Could you check a few things on this model? Use its own coordinates, in mm. Face numbers are marked on the shaded views. A direction names the side the tool comes from. Give positions to 0.01 mm unless a question says otherwise; leave off trailing zeros. Order: outer loops, then holes, each group sorted by start corner. A loop starts at its lowest first (then second) coordinate and runs counter-clockwise, first axis right, second up. Notation, with made-up numbers: (-39, 18) - (13, 18) arc R25 ccw to (13, 47) - close; hole circle Ø5 at (47.25, 71.25). An arc over 180 degrees is marked (long way). Put each result on its own line as item: value.
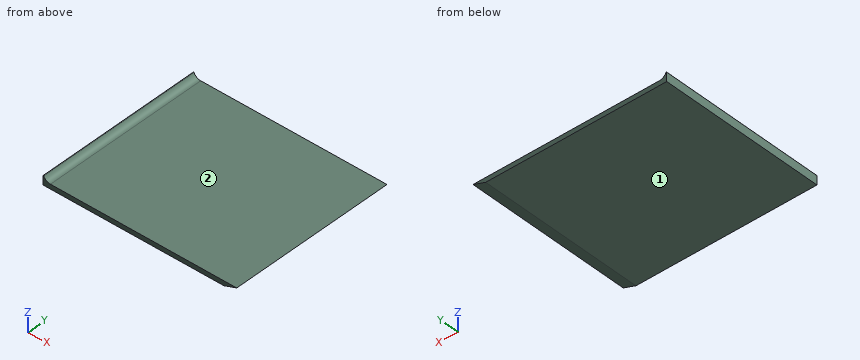
from build123d import *

# Parameters (mm, degrees)
SKETCH1_W           = 195
SKETCH1_H           = 180
BOSS_EXTRUDE1_DEPTH = 2.5
BOSS_EXTRUDE3_DEPTH = 180
BOSS_EXTRUDE4_DEPTH = 180
FILLET1_R           = 0.4


with BuildPart() as part:
    # Sketch1 → Boss-Extrude1 (new body, symmetric)
    with BuildSketch(Plane.XY):
        Rectangle(SKETCH1_W, SKETCH1_H)
    extrude(amount=BOSS_EXTRUDE1_DEPTH, both=True)

    # Sketch4 → Boss-Extrude3 (add)
    with BuildSketch(Plane.XZ.offset(90)):
        with BuildLine():
            Line((-97.5, 2.5), (-97.5, 10.5))
            ThreePointArc((-97.5, 10.5), (-95.156854249, 4.843145751), (-89.5, 2.5))
            Line((-89.5, 2.5), (-97.5, 2.5))
        make_face()
    extrude(amount=-BOSS_EXTRUDE3_DEPTH)

    # Sketch5 → Boss-Extrude4 (add)
    with BuildSketch(Plane.XZ.offset(90)):
        Polygon((97.5, 2.5), (97.5, -2.5), (111.237387097, 2.5), align=None)
    extrude(amount=-BOSS_EXTRUDE4_DEPTH)

    # Fillet1
    fillet1_edges = [part.edges().sort_by_distance(p)[0] for p in [
        (-97.5, 0, 10.5),
    ]]
    fillet(fillet1_edges, radius=FILLET1_R)


solid = part.part
1) If I drill on line 1 (Z direction, x = -6, y = -13); line 2 (X direction, y = -16.5, z = 3.75); line 3 (X direction, y = 68.5, z = 4), over which ranges is the centre line in solid material (lowest first)? Write a range as [from, to].
Filled in:
line 1: z = [-2.5, 2.5]
line 2: x = [-97.5, -93.79]
line 3: x = [-97.5, -94.16]
2) Suppose I cut it at C-C, the plane z = 4.5. List the corners of the cut face in (x, y) for me.
Filled in:
outline: (-97.5, -90) - (-94.79, -90) - (-94.79, 90) - (-97.5, 90) - close
3) Suppose I cut it at B-B, the plane x = -26. List the corners of the cut face in (y, z) for me, and give its area (3 significant figures).
Filled in:
outline: (-90, -2.5) - (90, -2.5) - (90, 2.5) - (-90, 2.5) - close
area: 900 mm^2
4) Which directions (+Z, -Z, +X, -X, +Y, -Y) give clear straight access to the entire face, cutting with the end or side of a thin tool? Please do the marked faces 1 and 2.
Filled in:
face 1: -Z, +X, -X, +Y, -Y
face 2: +Z, +X, +Y, -Y
5) I'm going to push a flat-ended pin straight in: pin 1 (2 mm diameter, centred on x = 65.5, y = -20.5, fed in from +Z). Where does the tip first touch, or does it pass through?
Filled in:
pin 1: stops at z = 2.5
6) Suppose I cut it at A-A, the plane y = -62. List the corners of the cut face in (x, z) for me.
Filled in:
outline: (-97.5, -2.5) - (97.5, -2.5) - (111.24, 2.5) - (-89.5, 2.5) arc R8 cw to (-96.74, 7.09) arc R0.4 ccw to (-97.5, 6.92) - close
